Geometry check sheet. Reference: the model listing, model coordinates, mm. A direction names the side the tool comes from. Round coordinates to 2 decimals unless told otherwise and drop trailing zeros. Order: outer loops, then holes, each group sorted by start corner. A loop starts at its lowest first (then second) coordinate and runs counter-clockwise, first axis right, second up. Notation, with made-up numbers: (51, 3) - (60, 3) arc R26 cw to (60, 26) - close; hole circle Ø11 at (64.5, 22.5). An arc over 180 degrees is marked (long way). Write each question's results on one line, items separated by ' | '.
Autodesk Fusion 360 part; units mm, degrees
sketch "Sketch1" plane through (0, 0, 0) normal (0, 1, 0) x (1, 0, 0)
  circle A0 centre (0, 0) radius 11.1
  dimension "d1" = 22.2
extrude "Extrude1" add sketch "Sketch1" along normal blind 3.8
sketch "Sketch2" plane through (0, 0, 0) normal (0, -1, 0) x (1, 0, 0)
  circle A0 centre (0, 0) radius 11.1
  circle A1 centre (0, 0) radius 5.1
  dimension "d4" = 10.2
extrude "Extrude2" add sketch "Sketch2" along normal blind 9 contours A1
sketch "Sketch3" plane through (0, 3.8, 0) normal (0, 1, 0) x (-1, 0, 0)
  circle A0 centre (0, 0) radius 11.1
  circle A1 centre (0, 0) radius 5.1
  dimension "d7" = 10.2
extrude "Extrude3" add sketch "Sketch3" along normal blind 2 contours A1
sketch "Sketch4" plane through (0, 5.8, 0) normal (0, 1, 0) x (-1, 0, 0)
  circle A0 centre (0, 0) radius 5.1
  circle A1 centre (0, 0) radius 4
  dimension "d10" = 8
extrude "Extrude4" cut sketch "Sketch4" against normal blind 17 contours A1
sketch "Sketch5" plane through (0, 0, 0) normal (0, -1, 0) x (1, 0, 0)
  circle A0 centre (0, 0) radius 5.1
  circle A1 centre (0, 0) radius 11.1
  circle A2 centre (0, 0) radius 8
  circle A3 centre (-8, 0) radius 1.75
  line L0 (0, 0) -> (-16, 0)
  line L1 (-16, 0) -> (-16, 13)
  line L2 (-16, 13) -> (0, 13)
  line L3 (0, 13) -> (0, 0)
  line L4 (0, 0) -> (14, 0)
  line L5 (14, 0) -> (14, -12)
  line L6 (14, -12) -> (0, -12)
  line L7 (0, -12) -> (0, 0)
  circle A4 centre (0, 8) radius 1.75
  circle A5 centre (0, -8) radius 1.75
  circle A6 centre (8, 0) radius 1.75
  dimension "d13" = 16
  dimension "d14" = 3.5
  dimension "d15" = 3.5
  dimension "d16" = 3.5
  dimension "d17" = 3.5
extrude "Extrude5" cut sketch "Sketch5" against normal blind 7 contours A2 L4 A6 | A2 L4 A6 | A2 L3 A4 | A2 L3 A4 | A2 L7 A5 | A2 L7 A5 | A2 L4 A6 | A2 L4 A6 | A2 A3 L0 | A2 A3 L0 | A2 L3 A4 | A2 L3 A4 | A2 L7 A5 | A2 L7 A5 | A2 A3 L0 | A2 A3 L0
(1) Material ranges on line 1 (Z direction, x = 0, y = 2.95); line 2 (Y direction, x = -7, z = 2.75); line 3 (Z direction, x = -8, y = 2.55), recorded low to high.
Answers follow:
line 1: -11.1 to -9.75, -6.25 to -4, 4 to 6.25, 9.75 to 11.1 | line 2: 0 to 3.8 | line 3: -7.69 to -1.75, 1.75 to 7.69
(2) Depth check by flat-ended pin: pin 1 Ø4 at (x, y) = (3.5, -1.5) entering from -Z; pin 2 Ø1 at (y, z) = (3, 3.5) entering from +X; pin 3 Ø5 at (x, z) = (-6, 4) entering from +Y; pin 4 Ø1.5 at (y, z) = (-1, -2) entering from +X. Enter the tip coordinate at first touch or a pass-through.
Answers follow:
pin 1: z = -10.88 | pin 2: x = 10.69 | pin 3: y = 5.8 | pin 4: x = 4.94
(3) Section check B-B (z = 0). Record the cut outline in (x, y).
Answers follow:
outline: (-11.1, 0) - (-9.75, 0) - (-9.75, 3.8) - (-11.1, 3.8) - close; (-6.25, 0) - (-5.1, 0) - (-5.1, -9) - (-4, -9) - (-4, 5.8) - (-5.1, 5.8) - (-5.1, 3.8) - (-6.25, 3.8) - close; (4, -9) - (5.1, -9) - (5.1, 0) - (6.25, 0) - (6.25, 3.8) - (5.1, 3.8) - (5.1, 5.8) - (4, 5.8) - close; (9.75, 0) - (11.1, 0) - (11.1, 3.8) - (9.75, 3.8) - close
(4) Access from +Z, -Z, +X, -X, +Y, -Y to the whole of each face (thin tool, end or side, straight path). Record for faces 1 (the face through (2.4, -4.4, 4.5)), 2 (the face through (0.867, -1.496, -3.905)), 3 (the face through (-2.4, 4.8, 4.5)).
Answers follow:
face 1: -Y | face 2: +Y, -Y | face 3: +Y
(5) Draft check along Z on faces 4 (the face through (5.97, 1.87, 9.36)), 5 (the face through (2, 0, 5)), 6 (the face through (1.617, 1.873, -8.67)). Enter one of: released by +Z, released by -Z, zero draft, split by the parting line, or undercut.
Answers follow:
face 4: split by the parting line | face 5: zero draft | face 6: undercut
(6) Section check D-D (z = 9). Record the cut outline in (x, y).
Answers follow:
outline: (-6.5, 0) - (-1.44, 0) - (-1.44, 3.8) - (-6.5, 3.8) - close; (1.44, 0) - (6.5, 0) - (6.5, 3.8) - (1.44, 3.8) - close
(7) Section check C-C (y = 3.25). Record the cut outline in (x, z), then the cut area to 3 significant figures.
Answers follow:
outline: circle Ø22.2 at (0, 0); hole circle Ø3.5 at (-8, 0); hole circle Ø8 at (0, 0); hole circle Ø3.5 at (0, -8); hole circle Ø3.5 at (0, 8); hole circle Ø3.5 at (8, 0) | area: 298 mm²
(8) Section check A-A (x = 0). Record the cut outline in (y, z), then the cut area to 3 significant figures.
Answers follow:
outline: (-9, -5.1) - (0, -5.1) - (0, -6.25) - (3.8, -6.25) - (3.8, -5.1) - (5.8, -5.1) - (5.8, -4) - (-9, -4) - close; (-9, 4) - (5.8, 4) - (5.8, 5.1) - (3.8, 5.1) - (3.8, 6.25) - (0, 6.25) - (0, 5.1) - (-9, 5.1) - close; (0, -11.1) - (3.8, -11.1) - (3.8, -9.75) - (0, -9.75) - close; (0, 9.75) - (3.8, 9.75) - (3.8, 11.1) - (0, 11.1) - close | area: 51.6 mm²
